Here's how the part is built. I have some questions about the finished solid (model axes, mm). Coordinates: 2 decimals unless noted, no trailing zeros. Loops run counter-clockwise (first coordinate to the right, second up) from the corner with the lowest first, then second, coordinate; pieces in that order, holes last. Notation, with made-up numbers: M -38.75,63.25 L 12.25,63.25 A17 cw 12.25,93.25 Z; hole C 64,14 d8. An arc over 180 degrees is marked long. Use one line per item in the form item = value. Start each with the question number.
(1) Imagine slicing it at A-A, the plane y = 3. State how many separate pieces and enclosed holes the cut face has, and give its area (3 significant figures).
(2) Will this pin go through, and if not, where does the flat tip stop? P1, Ø1.7, axis at x = 113.03, z = -111.18, coming from the -Y side.
(3) Imagine slicing it at B-B, the plane z = -142.5. Please give me the cut outline in (x, y), and give its area (3 significant figures).
(4) Please list where these lines run through material, in increasing order: L1, parallel to X at y = 3.75, z = -251.5; L2, parallel to Z at x = 125.73, y = 2; L3, parallel to Z at x = 69.85, y = 4.5.
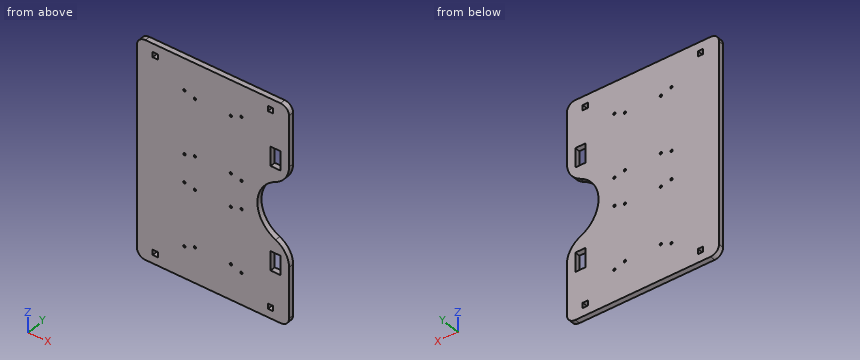
```python
from build123d import *

# Parameters (mm, degrees)
SKETCH3_R           = 1.4224
SKETCH3_W           = 6.35
SKETCH3_H           = 6.35
SKETCH3_W_2         = 11.938
SKETCH3_H_2         = 23.114
BOSS_EXTRUDE1_DEPTH = 6.35
FILLET1_R           = 10.16
FILLET2_R           = 27.94


with BuildPart() as part:
    # Sketch3 → Boss-Extrude1 (new body)
    with BuildSketch(Plane(origin=(0, 0, 0), x_dir=(1, 0, 0), z_dir=(0, 1, 0))):
        with BuildLine():
            Line((182.88, 0), (0, 0))
            Line((0, 0), (0, 262.339276313))
            Line((0, 262.339276313), (182.88, 262.339276313))
            Line((182.88, 262.339276313), (182.88, 169.269638157))
            ThreePointArc((182.88, 169.269638157), (144.78, 131.169638157), (182.88, 93.069638157))
            Line((182.88, 93.069638157), (182.88, 0))
        make_face()
        with Locations(Location((57.15, 38.1, 0), (0, 0, 270))):
            Circle(SKETCH3_R, mode=Mode.SUBTRACT)
        with Locations(Location((57.15, 114.3, 0), (0, 0, 270))):
            Circle(SKETCH3_R, mode=Mode.SUBTRACT)
        with Locations(Location((125.73, 114.3, 0), (0, 0, 90))):
            Circle(SKETCH3_R, mode=Mode.SUBTRACT)
        with Locations(Location((125.73, 38.1, 0), (0, 0, 90))):
            Circle(SKETCH3_R, mode=Mode.SUBTRACT)
        with Locations(Location((69.85, 151.157668748, 0), (0, 0, 270))):
            Circle(SKETCH3_R, mode=Mode.SUBTRACT)
        with Locations(Location((69.85, 219.737668748, 0), (0, 0, 270))):
            Circle(SKETCH3_R, mode=Mode.SUBTRACT)
        with Locations(Location((113.03, 151.157668748, 0), (0, 0, 90))):
            Circle(SKETCH3_R, mode=Mode.SUBTRACT)
        with Locations(Location((113.03, 219.737668748, 0), (0, 0, 90))):
            Circle(SKETCH3_R, mode=Mode.SUBTRACT)
        with Locations(Location((113.03, 42.601607565, 0), (0, 0, 270))):
            Circle(SKETCH3_R, mode=Mode.SUBTRACT)
        with Locations(Location((113.03, 111.181607565, 0), (0, 0, 270))):
            Circle(SKETCH3_R, mode=Mode.SUBTRACT)
        with Locations(Location((69.85, 111.181607565, 0), (0, 0, 90))):
            Circle(SKETCH3_R, mode=Mode.SUBTRACT)
        with Locations(Location((69.85, 42.601607565, 0), (0, 0, 90))):
            Circle(SKETCH3_R, mode=Mode.SUBTRACT)
        with Locations(Location((125.73, 148.039276313, 0), (0, 0, 270))):
            Circle(SKETCH3_R, mode=Mode.SUBTRACT)
        with Locations(Location((125.73, 224.239276313, 0), (0, 0, 270))):
            Circle(SKETCH3_R, mode=Mode.SUBTRACT)
        with Locations(Location((57.15, 224.239276313, 0), (0, 0, 90))):
            Circle(SKETCH3_R, mode=Mode.SUBTRACT)
        with Locations(Location((57.15, 148.039276313, 0), (0, 0, 90))):
            Circle(SKETCH3_R, mode=Mode.SUBTRACT)
        with Locations((22.225, 13.212735966)):
            Rectangle(SKETCH3_W, SKETCH3_H, mode=Mode.SUBTRACT)
        with Locations((160.655, 13.212735966)):
            Rectangle(SKETCH3_W, SKETCH3_H, mode=Mode.SUBTRACT)
        with Locations((160.655, 249.126540348)):
            Rectangle(SKETCH3_W, SKETCH3_H, mode=Mode.SUBTRACT)
        with Locations((22.225, 249.126540348)):
            Rectangle(SKETCH3_W, SKETCH3_H, mode=Mode.SUBTRACT)
        with Locations((166.751, 193.526638157)):
            Rectangle(SKETCH3_W_2, SKETCH3_H_2, mode=Mode.SUBTRACT)
        with Locations((166.751, 68.812638157)):
            Rectangle(SKETCH3_W_2, SKETCH3_H_2, mode=Mode.SUBTRACT)
    extrude(amount=BOSS_EXTRUDE1_DEPTH)

    # Fillet1
    fillet1_edges = [part.edges().sort_by_distance(p)[0] for p in [
        (0, 3.175, -262.339276313),
        (182.88, 3.175, -262.339276313),
        (182.88, 3.175, 0),
        (0, 3.175, 0),
    ]]
    fillet(fillet1_edges, radius=FILLET1_R)

    # Fillet2
    fillet2_edges = [part.edges().sort_by_distance(p)[0] for p in [
        (182.88, 3.175, -169.269638157),
        (182.88, 3.175, -93.069638157),
    ]]
    fillet(fillet2_edges, radius=FILLET2_R)


solid = part.part
```
Answer:
q1.separate_pieces = 1
q1.enclosed_holes = 22
q1.area = 44,600 mm²
q2.P1 = through
q3.outline = M 0,0 L 146.5,0 L 146.5,6.35 L 0,6.35 Z
q3.area = 930 mm²
q4.L1 = 0 to 19.05, 25.4 to 157.48, 163.83 to 182.88
q4.L2 = -262.34 to -225.66, -222.82 to -149.46, -146.62 to -115.72, -112.88 to -39.52, -36.68 to 0
q4.L3 = -262.34 to -221.16, -218.32 to -152.58, -149.74 to -112.6, -109.76 to -44.02, -41.18 to 0
